```python
from build123d import *

# Parameters (mm, degrees)
BOSS_EXTRUDE1_DEPTH = 6
FILLET1_R           = 10
SKETCH2_R           = 2.5
CUT_EXTRUDE1_DEPTH  = 6
SKETCH8_W           = 16
SKETCH8_H           = 121.699623713
CUT_EXTRUDE5_DEPTH  = 2
SKETCH9_R           = 15
CUT_EXTRUDE6_DEPTH  = 4
SKETCH10_R          = 4.460390543
BOSS_EXTRUDE2_DEPTH = 2
FILLET2_R           = 10
SKETCH12_R          = 1.5
CUT_EXTRUDE7_DEPTH  = 10
SKETCH13_R          = 1.5
CUT_EXTRUDE8_DEPTH  = 10
SKETCH14_R          = 2
CUT_EXTRUDE9_DEPTH  = 10


with BuildPart() as part:
    # Sketch1 → Boss-Extrude1 (new body)
    with BuildSketch(Plane(origin=(0, 0, 0), x_dir=(1, 0, 0), z_dir=(0, 1, 0))):
        Polygon((21.213083016, -102.227633762), (35.213083016, -90.480238926), (35.213083016, -30.480238926), (21.213083016, -18.73284409), (21.213083016, 31.26715591), (35.213083016, 43.014550747), (35.213083016, 103.014550747), (-36.786916984, 103.014550747), (-36.786916984, 43.014550747), (-22.786916984, 31.26715591), (-22.786916984, -18.73284409), (-36.786916984, -30.480238926), (-36.786916984, -90.480238926), (-22.786916984, -102.227633762), align=None)
    extrude(amount=BOSS_EXTRUDE1_DEPTH)

    # Fillet1
    fillet1_edges = [part.edges().sort_by_distance(p)[0] for p in [
        (-22.786916984, 3, 102.227633762),
        (-36.786916984, 3, 90.480238926),
        (-36.786916984, 3, 30.480238926),
        (-22.786916984, 3, 18.73284409),
        (21.213083016, 3, 18.73284409),
        (35.213083016, 3, 30.480238926),
        (35.213083016, 3, 90.480238926),
        (21.213083016, 3, 102.227633762),
    ]]
    fillet(fillet1_edges, radius=FILLET1_R)

    # Sketch2 → Cut-Extrude1 (cut)
    with BuildSketch(Plane.XZ):
        with Locations(Location((-0.786916984, 60.480238926, 0), (0, 0, 270))):
            Circle(SKETCH2_R)
    extrude(amount=-CUT_EXTRUDE1_DEPTH, mode=Mode.SUBTRACT)

    # Sketch8 → Cut-Extrude5 (cut)
    with BuildSketch(Plane(origin=(0, 6, 0), x_dir=(1, 0, 0), z_dir=(0, 1, 0))):
        with Locations((-0.786916984, 9.974259286)):
            Rectangle(SKETCH8_W, SKETCH8_H)
    extrude(amount=-CUT_EXTRUDE5_DEPTH, mode=Mode.SUBTRACT)

    # Sketch9 → Cut-Extrude6 (cut)
    with BuildSketch(Plane(origin=(0, 6, 0), x_dir=(1, 0, 0), z_dir=(0, 1, 0))):
        with Locations(Location((-0.786916984, -60.480238926, 0), (0, 0, 270))):
            Circle(SKETCH9_R)
    extrude(amount=-CUT_EXTRUDE6_DEPTH, mode=Mode.SUBTRACT)

    # Sketch10 → Boss-Extrude2 (add)
    with BuildSketch(Plane(origin=(0, 2, 0), x_dir=(1, 0, 0), z_dir=(0, 1, 0))):
        with Locations((-0.786916984, -60.480238926)):
            Circle(SKETCH10_R)
    extrude(amount=-BOSS_EXTRUDE2_DEPTH)

    # Fillet2
    fillet2_edges = [part.edges().sort_by_distance(p)[0] for p in [
        (-22.786916984, 3, -31.26715591),
        (-36.786916984, 3, -43.014550747),
        (35.213083016, 3, -43.014550747),
        (21.213083016, 3, -31.26715591),
    ]]
    fillet(fillet2_edges, radius=FILLET2_R)

    # Sketch12 → Cut-Extrude7 (cut)
    with BuildSketch(Plane(origin=(0, 6, 0), x_dir=(1, 0, 0), z_dir=(0, 1, 0))):
        with Locations(Location((15.213083016, 6.26715591, 0), (0, 0, 270))):
            Circle(SKETCH12_R)
        with Locations(Location((-16.786916984, 6.26715591, 0), (0, 0, 270))):
            Circle(SKETCH12_R)
    extrude(amount=-CUT_EXTRUDE7_DEPTH, mode=Mode.SUBTRACT)

    # Sketch13 → Cut-Extrude8 (cut)
    with BuildSketch(Plane.XZ):
        with Locations(Location((-22.567416075, 90.043344962, 0), (0, 0, 270))):
            Circle(SKETCH13_R)
        with Locations(Location((20.993582106, 90.043344962, 0), (0, 0, 90))):
            Circle(SKETCH13_R)
    extrude(amount=-CUT_EXTRUDE8_DEPTH, mode=Mode.SUBTRACT)

    # Sketch14 → Cut-Extrude9 (cut)
    with BuildSketch(Plane.XZ):
        with Locations(Location((-26.786916984, -73.014550747, 0), (0, 0, 270))):
            Circle(SKETCH14_R)
        with Locations(Location((25.213083016, -73.014550747, 0), (0, 0, 270))):
            Circle(SKETCH14_R)
    extrude(amount=-CUT_EXTRUDE9_DEPTH, mode=Mode.SUBTRACT)


solid = part.part
```
Input: part model. Units: mm. Frame: model coordinates. A direction names the side the tool comes from. Give positions to 0.01 mm unless a question says otherwise; leave off trailing zeros. Loops run counter-clockwise (first coordinate to the right, second up) from the corner with the lowest first, then second, coordinate; pieces in that order, holes last. Notation, with made-up numbers: (32.5, 31) -> (53.5, 31) arc R8 ccw to (53.5, 37) -> close; hole circle Ø9 at (81, 3.5). An arc over 180 degrees is marked (long way). Use a Markdown table: item, result.
Q1. Section query B-B, the plane z = -20. Return the cut outline in (x, y).
Entries:
| item | result |
|---|---|
| outline | (-22.79, 0) -> (21.21, 0) -> (21.21, 6) -> (7.21, 6) -> (7.21, 4) -> (-8.79, 4) -> (-8.79, 6) -> (-22.79, 6) -> close |
Q2. Pull-direction query (Z, two-part tool) for faces 1 (the flat face through (-36.787, 3, 60)), 2 (the flat face through (-29.739, 2.958, 24.566)), 3 (the cylindrical face through (34.25, 3.04, 90.1)); classes: pulls with the +Z half, pulls with the -Z half, needs draft (parallel to the pull), parting line crosses it, or undercut.
Entries:
| item | result |
|---|---|
| face 1 | needs draft |
| face 2 | undercut |
| face 3 | pulls with the +Z half |
Q3. First-contact query: P1, Ø8, axis at x = 1, z = -4, coming from the +Y side; P2, Ø0.6, axis at y = 5, z = 1, coming from the +X side; P3, Ø2, axis at y = 3, z = -32, coming from the +X side; P4, Ø2.5, axis at x = -16.79, z = -6.27, coming from the -Y side. Flat tips, straight axial feed; report the tip coordinate or a pass-through.
Entries:
| item | result |
|---|---|
| P1 | stops at y = 4 |
| P2 | stops at x = 21.21 |
| P3 | stops at x = 23.53 |
| P4 | passes through |
Q4. Access query for faces 4 (the flat face through (-1, 2, 60)), 5 (the cylindrical face through (-23.7, 3.04, 18.24)), 6 (the cylindrical face through (34.25, 3.04, -43.4)). Directions: +Z, -Z, +X, -X, +Y, -Y. A direction counts if a zero-diameter tool reaches every point of the face in a straight line with its end or side. Return the directions, or none.
Entries:
| item | result |
|---|---|
| face 4 | +Y |
| face 5 | -X, +Y, -Y |
| face 6 | +X, +Y, -Y |
Q5. Section query A-A, the plane y = 3.1. State how many separate pieces and enclosed holes the cut face has, plus the area to 3 significant figures.
Entries:
| item | result |
|---|---|
| separate pieces | 1 |
| enclosed holes | 7 |
| area | 12,100 mm² |
Q6. Section query C-C, the plane x = -3. Return the cut outline in (y, z).
Entries:
| item | result |
|---|---|
| outline | (0, -103.01) -> (6, -103.01) -> (6, -70.82) -> (4, -70.82) -> (4, 45.64) -> (2, 45.64) -> (2, 75.32) -> (6, 75.32) -> (6, 102.23) -> (0, 102.23) -> close |
Q7. Section query D-D, the plane z = -69. Return the cut outline in (x, y), plus the area to 3 significant figures.
Entries:
| item | result |
|---|---|
| outline | (-36.79, 0) -> (35.21, 0) -> (35.21, 6) -> (7.21, 6) -> (7.21, 4) -> (-8.79, 4) -> (-8.79, 6) -> (-36.79, 6) -> close |
| area | 400 mm² |
Q8. Ray query, probe 1 along Z at (x, y) = (25.5, 4.6); probe 2 along Z at (x, y) = (24.5, 5.05); probe 3 along X at (y, z) = (4.4, -74). Return the intervals inside material, ascending. Write a range as from..to.
Entries:
| item | result |
|---|---|
| probe 1 | z = -103.01..-74.99, -71.04..-34.86, 22.33..98.63 |
| probe 2 | z = -103.01..-74.88, -71.15..-34.02, 21.48..99.47 |
| probe 3 | x = -36.79..-28.53, -25.05..23.47, 26.95..35.21 |
